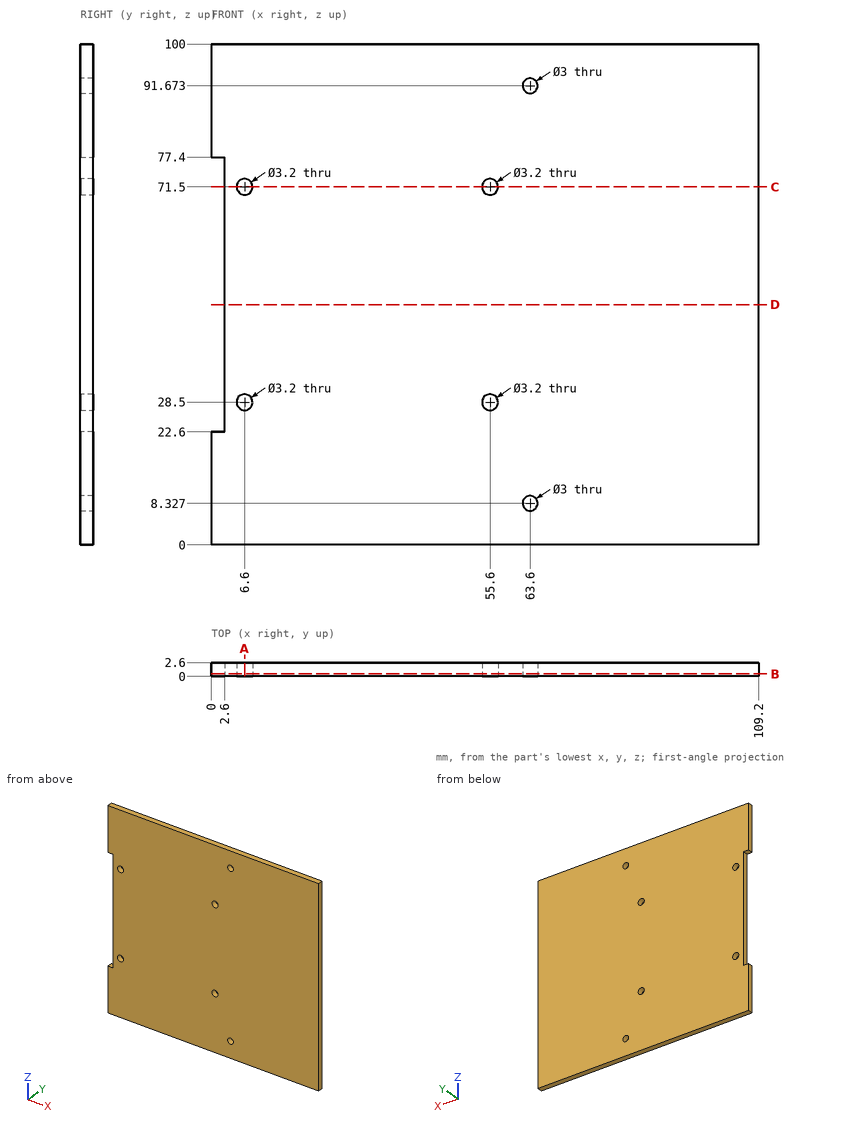
Could you check a few things on this drawing? It's one solid part, dimensions in mm from its lowest x, y, z. Give positions to 0.01 mm unless a question says otherwise; leave off trailing zeros. Write each loop counter-clockwise with the first axis right and the second up, starting at its lowest first coordinate (ties: lowest second). Pieces come first, ordered by that corner, then holes. Notation, with made-up numbers: (84.5, 4.5) -> (136.5, 4.5) arc R21 cw to (136.5, 31.5) -> close; hole circle Ø6 at (18.25, -6). An arc over 180 degrees is marked (long way). Write item = value, one per line.
(1) I need wall thicknesses on probe 1 along X at (y, z) = (1.1, 28.5); probe 2 along X at (y, z) = (2.3, 91.5); probe 3 along Z at (x, y) = (62.5, 1.15) (1 decimal). Which ranges of each line are inside material? Lowest first, please. Write a range as from..to.
Worked out:
probe_1 = 2.6..5, 8.2..54, 57.2..109.2
probe_2 = 0..62.11, 65.09..109.2
probe_3 = 0..7.3, 9.3..90.7, 92.7..100
(2) Suppose I cut it at A-A on x = 6.6. Write out the boundary of the cut face in (y, z).
Worked out:
outline = (0, 0) -> (2.6, 0) -> (2.6, 26.9) -> (0, 26.9) -> close; (0, 30.1) -> (2.6, 30.1) -> (2.6, 69.9) -> (0, 69.9) -> close; (0, 73.1) -> (2.6, 73.1) -> (2.6, 100) -> (0, 100) -> close
(3) Suppose I cut it at D-D on z = 48. Write out the boundary of the cut face in (x, y).
Worked out:
outline = (2.6, 0) -> (109.2, 0) -> (109.2, 2.6) -> (2.6, 2.6) -> close
(4) Suppose I cut it at B-B on y = 0.4. Write out the boundary of the cut face in (x, z), then the cut area to 3 significant figures.
Worked out:
outline = (0, 0) -> (109.2, 0) -> (109.2, 100) -> (0, 100) -> (0, 77.4) -> (2.6, 77.4) -> (2.6, 22.6) -> (0, 22.6) -> close; hole circle Ø3.2 at (6.6, 28.5); hole circle Ø3.2 at (6.6, 71.5); hole circle Ø3.2 at (55.6, 28.5); hole circle Ø3.2 at (55.6, 71.5); hole circle Ø3 at (63.6, 8.33); hole circle Ø3 at (63.6, 91.67)
area = 10,700 mm^2
(5) Suppose I cut it at C-C on z = 71.5. Write out the boundary of the cut face in (x, y).
Worked out:
outline = (2.6, 0) -> (5, 0) -> (5, 2.6) -> (2.6, 2.6) -> close; (8.2, 0) -> (54, 0) -> (54, 2.6) -> (8.2, 2.6) -> close; (57.2, 0) -> (109.2, 0) -> (109.2, 2.6) -> (57.2, 2.6) -> close
(6) I'm going to push a flat-ended pin straight in: P1, Ø0.8, axis at y = 0.5, z = 61.5, coming from the -X side. Where does the tip first touch, or does it pass through?
Worked out:
P1 = 2.6
